For this review, take the finished solid that the model builds, in its own axes (mm). A direction names the side the tool comes from. Give positions to 0.01 mm unless a question says otherwise; leave off trailing zeros. Write each loop counter-clockwise with the first axis right and the second up, starting at its lowest first coordinate (ties: lowest second). Pieces come first, ordered by that corner, then holes. Notation, with made-up numbers: M 25,41 L 79,41 A25 ccw 79,71 Z; hole C 4.5,16 d11. An arc over 180 degrees is marked long. One line per item, written item: value. Start each with the question number.
Item 1: Mouldability with a two-part tool opening along Y and no side actions: class faces 5 (the face through (9.468, -3.926, 1.726)), 6 (the face through (9, 2.499, 1)), 7 (the face through (0.1, 5.5, 0.9)), 8 (the face through (-1, 7, 1.7)) as released by +Y, released by -Y, zero draft, split by the parting line, or undercut.
Item 2: Consider section D-D, the plane y = -7.5. Write out the cut boundary in (x, z).
Item 3: Consider section A-A, the plane x = 0. Write out the cut boundary in (y, z).
Item 4: To check wall thickness, follow probe 1 along Y at (x, z) = (0, 3); probe 2 along Y at (x, z) = (0, 1.05); probe 3 along Y at (x, z) = (-8.75, 1.35). State the ranges of each line that lie inside material, in increasing order.
Item 5: Clearance check with flat-ended pins moving along their axes: pin 1 Ø1.4 at (y, z) = (8.5, 0.5) entering from +X; pin 2 Ø1.4 at (x, z) = (8.5, 1) entering from -Y; pin 3 Ø4 at (x, y) = (-0.5, -7.5) entering from -Z; pin 4 Ø0.5 at (x, z) = (8.5, 0.5) entering from +Y. State where each tip first meets the part, or that it passes through.
Item 6: Consider section C-C, the plane z = 1.45. Write out the cut boundary in (x, y), and give its area (3 significant figures).
Item 7: Tool access review of faces 1 (the face through (2.5, 9, 1)), 2 (the face through (7, -1, 1.7)), 3 (the face through (-9.4, 0, 1.7)), 4 (the face through (2.498, -9, 1)): name each direction out of +Z, -Z, +X, -X, +Y, -Y from which nothing blocks a thin tool from reaching the whole face with its end or side.
```python
from build123d import *

# Parameters (mm, degrees)
SKETCH1_R              = 10.25
SKETCH1_R_2            = 2
SKETCH1_R_3            = 1.2
BOSS_EXTRUDE1_DEPTH    = 3.5
CUT_EXTRUDE2_START     = -1.7
CUT_EXTRUDE2_OUTLINE_R = 1.2
CUT_EXTRUDE2_DEPTH     = 1.7


# Read off the part's stored shape, not the designer's step: Cut-Extrude2
with BuildPart() as part:
    # Sketch1 → Boss-Extrude1 (new body)
    with BuildSketch(Plane.XY):
        Circle(SKETCH1_R)
        Circle(SKETCH1_R_2, mode=Mode.SUBTRACT)
        with Locations((0, 8)):
            Circle(SKETCH1_R_3, mode=Mode.SUBTRACT)
        with Locations((8, 0)):
            Circle(SKETCH1_R_3, mode=Mode.SUBTRACT)
        with Locations((0, -8)):
            Circle(SKETCH1_R_3, mode=Mode.SUBTRACT)
        with Locations((-8, 0)):
            Circle(SKETCH1_R_3, mode=Mode.SUBTRACT)
    extrude(amount=BOSS_EXTRUDE1_DEPTH)

    # Cut-Extrude2 outline → Cut-Extrude2 (cut)
    # profile 1 of 4: a face of its own
    with BuildSketch(Plane(origin=(0, 0, 0), x_dir=(-1, 0, 0), z_dir=(0, 0, -1)).offset(CUT_EXTRUDE2_START)):
        with BuildLine():
            Line((-9.94069912, -2.499), (-8.098979998, -2.499))
            ThreePointArc((-8.098979998, -2.499), (-5.49948025, -0.050000196), (-8.000999999, 2.4989992))
            Line((-8.000999999, 2.4989992), (-9.940699321, 2.4989992))
            ThreePointArc((-9.940699321, 2.4989992), (-10.25, -4.12e-07), (-9.94069912, -2.499))
        make_face()
        with Locations((-8, 0)):
            Circle(CUT_EXTRUDE2_OUTLINE_R, mode=Mode.SUBTRACT)
    # profile 2 of 4: a face of its own
    with BuildSketch(Plane(origin=(0, 0, 0), x_dir=(-1, 0, 0), z_dir=(0, 0, -1)).offset(CUT_EXTRUDE2_START)):
        with BuildLine():
            Line((-2.498, -8), (-2.498, -9.940950458))
            ThreePointArc((-2.498, -9.940950458), (0.001546691, -10.249999883), (2.501, -9.940196125))
            Line((2.501, -9.940196125), (2.5010004, -8.070689462))
            ThreePointArc((2.5010004, -8.070689462), (0.037348265, -5.500249912), (-2.498, -8))
        make_face()
        with Locations((0, -8)):
            Circle(CUT_EXTRUDE2_OUTLINE_R, mode=Mode.SUBTRACT)
    # profile 3 of 4: a face of its own
    with BuildSketch(Plane(origin=(0, 0, 0), x_dir=(-1, 0, 0), z_dir=(0, 0, -1)).offset(CUT_EXTRUDE2_START)):
        with BuildLine():
            ThreePointArc((2.5, 9.940447676), (0, 10.25), (-2.5, 9.940447676))
            Line((-2.5, 9.940447676), (-2.5, 8))
            ThreePointArc((-2.5, 8), (0, 5.5), (2.5, 8))
            Line((2.5, 8), (2.5, 9.940447676))
        make_face()
        with Locations((0, 8)):
            Circle(CUT_EXTRUDE2_OUTLINE_R, mode=Mode.SUBTRACT)
    # profile 4 of 4: a face of its own
    with BuildSketch(Plane(origin=(0, 0, 0), x_dir=(-1, 0, 0), z_dir=(0, 0, -1)).offset(CUT_EXTRUDE2_START)):
        with BuildLine():
            Line((8.001, -2.499), (9.94069912, -2.499))
            ThreePointArc((9.94069912, -2.499), (10.249999948, 0.001031141), (9.940196125, 2.501))
            Line((9.940196125, 2.501), (8.001, 2.501))
            ThreePointArc((8.001, 2.501), (5.501, 0.001), (8.001, -2.499))
        make_face()
        with Locations((8, 0)):
            Circle(CUT_EXTRUDE2_OUTLINE_R, mode=Mode.SUBTRACT)
    extrude(amount=CUT_EXTRUDE2_DEPTH, mode=Mode.SUBTRACT)


solid = part.part
```
Model answer:
1. face 5: split by the parting line
1. face 6: undercut
1. face 7: released by +Y
1. face 8: zero draft
2. outline: M -6.99,0 L -2.45,0 L -2.45,1.7 L -1.09,1.7 L -1.09,3.5 L -6.99,3.5 Z; M 1.09,1.7 L 2.45,1.7 L 2.45,0 L 6.99,0 L 6.99,3.5 L 1.09,3.5 Z
3. outline: M -10.25,1.7 L -9.2,1.7 L -9.2,3.5 L -10.25,3.5 Z; M -6.8,1.7 L -5.5,1.7 L -5.5,0 L -2,0 L -2,3.5 L -6.8,3.5 Z; M 2,0 L 5.5,0 L 5.5,1.7 L 6.8,1.7 L 6.8,3.5 L 2,3.5 Z; M 9.2,1.7 L 10.25,1.7 L 10.25,3.5 L 9.2,3.5 Z
4. probe 1: y = -10.25 to -9.2, -6.8 to -2, 2 to 6.8, 9.2 to 10.25
4. probe 2: y = -5.5 to -2, 2 to 5.5
4. probe 3: y = -5.34 to -2.5, 2.5 to 5.34
5. pin 1: stops at x = 6.65
5. pin 2: stops at y = -6.65
5. pin 3: stops at z = 0
5. pin 4: stops at y = 6.08
6. outline: M -9.94,-2.5 A10.25 ccw -2.5,-9.94 L -2.5,-8.07 A2.5 cw long 2.5,-8 L 2.5,-9.94 A10.25 ccw 9.94,-2.5 L 8.1,-2.5 A2.5 cw long 8,2.5 L 9.94,2.5 A10.25 ccw 2.5,9.94 L 2.5,8 A2.5 cw -2.5,8 L -2.5,9.94 A10.25 ccw -9.94,2.5 L -8,2.5 A2.5 cw -8,-2.5 Z; hole C 0,0 d4
6. area: 235 mm2
7. face 1: -Z, +Y
7. face 2: -Z, +X
7. face 3: -Z, -X
7. face 4: -Z, -Y
